```python
from build123d import *

# Parameters (mm, degrees)
SKETCH1_W           = 139.7
SKETCH1_H           = 25.4
BOSS_EXTRUDE1_DEPTH = 3.175
SKETCH2_R           = 4.7625
CUT_EXTRUDE1_DEPTH  = 7.35


with BuildPart() as part:
    # Sketch1 → Boss-Extrude1 (new body, symmetric)
    with BuildSketch(Plane(origin=(0, 0, 0), x_dir=(1, 0, 0), z_dir=(0, 1, 0))):
        Rectangle(SKETCH1_W, SKETCH1_H)
    extrude(amount=BOSS_EXTRUDE1_DEPTH, both=True)

    # Sketch2 → Cut-Extrude1 (cut, through all)
    with BuildSketch(Plane(origin=(0, 3.175, 0), x_dir=(1, 0, 0), z_dir=(0, 1, 0))):
        with Locations((50.8, 0)):
            Circle(SKETCH2_R)
        with Locations((-50.8, 0)):
            Circle(SKETCH2_R)
    extrude(amount=-CUT_EXTRUDE1_DEPTH, mode=Mode.SUBTRACT)


solid = part.part
```
The listing builds one solid part. Answer for the finished solid, in the listing's coordinates (mm). Give positions to 0.01 mm unless a question says otherwise; leave off trailing zeros. Order: outer loops, then holes, each group sorted by start corner. A loop starts at its lowest first (then second) coordinate and runs counter-clockwise, first axis right, second up.
Item 1: For a pull along Z with two mould halves and no side action, classify faces 1 (the face through (-1, 0, -12.7)), 2 (the face through (-1, 3.175, 0)), 3 (the face through (46.042, 0.044, -0.209)) as pulls with the +Z half, pulls with the -Z half, needs draft (parallel to the pull), parting line crosses it, or undercut.
From the geometry:
face 1: pulls with the -Z half
face 2: needs draft
face 3: undercut
Item 2: The part is cut by section A-A, the plane y = 2. Count the separate pieces of the cut face and the enclosed holes in it, and give its area (3 significant figures).
From the geometry:
separate pieces: 1
enclosed holes: 2
area: 3,410 mm2
Item 3: Find the intervals of material crossed by probe 1 along X at (y, z) = (1.5, 0); probe 2 along Z at (x, y) = (50.8, 1.5); probe 3 along X at (y, z) = (1.25, -2), in increasing order.
From the geometry:
probe 1: x = -69.85 to -55.56, -46.04 to 46.04, 55.56 to 69.85
probe 2: z = -12.7 to -4.76, 4.76 to 12.7
probe 3: x = -69.85 to -55.12, -46.48 to 46.48, 55.12 to 69.85
Item 4: Given pin 1 Ø7.5 at (x, z) = (50.8, 0) entering from -Y, flat-ended and moving along its own axis, determine where the tip first touches the part or whether it passes through.
From the geometry:
pin 1: passes through
Item 5: The part is cut by section B-B, the plane x = -50.8. Give the vertices of the cut face in (y, z) (1 decimal), and give its area (3 significant figures).
From the geometry:
outline: (-3.2, -12.7) - (3.2, -12.7) - (3.2, -4.8) - (-3.2, -4.8) - close; (-3.2, 4.8) - (3.2, 4.8) - (3.2, 12.7) - (-3.2, 12.7) - close
area: 101 mm2
